Part model, mm, in its own coordinate system. A direction names the side the tool comes from. Coordinates: 2 decimals unless noted, no trailing zeros. Write each loop counter-clockwise with the first axis right and the second up, starting at its lowest first coordinate (ties: lowest second). Pieces come first, ordered by that corner, then holes. Notation, with made-up numbers: M 24.25,-19 L 30.25,-19 A20 ccw 30.25,10 Z; hole C 13.5,48.25 d10. An arc over 180 degrees is marked long. Use a Markdown table: item, result. Add a question column.
Q1. Pin check, flat tips, straight feed: pin 1 Ø4 at (y, z) = (56, -7) entering from -X; pin 2 Ø2 at (y, z) = (58, -27.5) entering from -X; pin 3 Ø10 at (y, z) = (73, 30.5) entering from -X. Stop position of each tip, or through.
Q2. Slice it at C-C on x = 0. Write the cut outline in (y, z).
Q3. Slice it at D-D on z = -47.5. Write the cut outline in (x, y).
Q4. Wall check: L1, parallel to X at y = 67, z = 0; L2, parallel to X at y = 39, z = -31.5. Give the ranges that are in metal, low to high. Write a range as from..to.
Q5. Slice it at A-A on y = 30. Write the cut outline in (x, z), then the cut area to 3 significant figures.
Q6. Tool access for faces 1 (the cylindrical face through (0.7, 55.594, -55.719)), 2 (the cylindrical face through (-28, 75, 21)), 3 (the cylindrical face through (57.15, 25.35, -56.99)): list every direction of +Z, -Z, +X, -X, +Y, -Y with a clear straight run to the whole face (end or side of a thin tool).
Q7. Slice it at B-B on z = 0. Write the cut outline in (x, y).
Q8. Mould opens along X. For faces 4 (the cylindrical face through (-57.15, 25.35, 56.99)), 5 (the flat face through (-1, 25, 60)), 6 (the flat face through (-1, 25, 58)) say: released by +X, released by -X, zero draft, split by the parting line, or undercut.
from build123d import *

# Parameters (mm, degrees)
CROQUIS2_W              = 120
CROQUIS2_H              = 120
SALIENTE_EXTRUIR1_DEPTH = 60
REDONDEO1_R             = 10
VACIADO1_T              = -2
CROQUIS3_R              = 35
SALIENTE_EXTRUIR2_DEPTH = 25
CROQUIS4_R              = 25
CORTAR_EXTRUIR1_DEPTH   = 86
REDONDEO2_R             = 5


with BuildPart() as part:
    # Croquis2 → Saliente-Extruir1 (new body)
    with BuildSketch(Plane(origin=(0, 0, 0), x_dir=(1, 0, 0), z_dir=(0, 1, 0))):
        Rectangle(CROQUIS2_W, CROQUIS2_H)
    extrude(amount=SALIENTE_EXTRUIR1_DEPTH)

    # Redondeo1
    redondeo1_edges = [part.edges().sort_by_distance(p)[0] for p in [
        (-60, 60, 0),
        (0, 60, 60),
        (60, 60, 0),
        (60, 30, 60),
        (-60, 30, 60),
        (-60, 30, -60),
        (60, 30, -60),
        (0, 60, -60),
    ]]
    fillet(redondeo1_edges, radius=REDONDEO1_R)

    # Vaciado1
    vaciado1_openings = [part.faces().sort_by_distance(p)[0] for p in [
        (0, 0, 0),
    ]]
    offset(amount=VACIADO1_T, openings=vaciado1_openings, kind=Kind.INTERSECTION)

    # Croquis3 → Saliente-Extruir2 (add)
    with BuildSketch(Plane(origin=(0, 60, 0), x_dir=(1, 0, 0), z_dir=(0, 1, 0))):
        Circle(CROQUIS3_R)
    extrude(amount=SALIENTE_EXTRUIR2_DEPTH)

    # Croquis4 → Cortar-Extruir1 (cut, through all)
    with BuildSketch(Plane(origin=(0, 85, 0), x_dir=(1, 0, 0), z_dir=(0, 1, 0))):
        Circle(CROQUIS4_R)
    extrude(amount=-CORTAR_EXTRUIR1_DEPTH, mode=Mode.SUBTRACT)

    # Redondeo2
    redondeo2_edges = [part.edges().sort_by_distance(p)[0] for p in [
        (-35, 60, 0),
    ]]
    fillet(redondeo2_edges, radius=REDONDEO2_R)


solid = part.part
Recorded:
| question | item | result |
|---|---|---|
| 1 | pin 1 | x = -59.17 |
| 1 | pin 2 | x = -57.14 |
| 1 | pin 3 | x = -23.97 |
| 2 | outline | M 0,-60 L 50,-60 A10 ccw 60,-50 L 60,-40 A5 cw 65,-35 L 85,-35 L 85,-25 L 58,-25 L 58,-50 A8 cw 50,-58 L 0,-58 Z; M 0,58 L 50,58 A8 cw 58,50 L 58,25 L 85,25 L 85,35 L 65,35 A5 cw 60,40 L 60,50 A10 ccw 50,60 L 0,60 Z |
| 3 | outline | M -60,0 L -58,0 L -58,50 A8 cw -50,58 L 50,58 A8 cw 58,50 L 58,0 L 60,0 L 60,50 A10 ccw 50,60 L -50,60 A10 ccw -60,50 Z |
| 4 | L1 | -35..-25, 25..35 |
| 4 | L2 | -60..-58, 58..60 |
| 5 | outline | M -60,-50 A10 ccw -50,-60 L 50,-60 A10 ccw 60,-50 L 60,50 A10 ccw 50,60 L -50,60 A10 ccw -60,50 Z; hole M -58,-50 A8 ccw -50,-58 L 50,-58 A8 ccw 58,-50 L 58,50 A8 ccw 50,58 L -50,58 A8 ccw -58,50 Z |
| 5 | area | 913 mm² |
| 6 | face 1 | -Y |
| 6 | face 2 | +Y |
| 6 | face 3 | -Z, +X, +Y, -Y |
| 7 | outline | M -60,0 L -58,0 L -58,50 A8 cw -50,58 L -25,58 L -25,85 L -35,85 L -35,65 A5 cw -40,60 L -50,60 A10 ccw -60,50 Z; M 25,58 L 50,58 A8 cw 58,50 L 58,0 L 60,0 L 60,50 A10 ccw 50,60 L 40,60 A5 cw 35,65 L 35,85 L 25,85 Z |
| 8 | face 4 | released by -X |
| 8 | face 5 | zero draft |
| 8 | face 6 | undercut |
